Answer from the drawing. Dimensions are ordinates in mm from the lowest x, y and z of the part. Give positions to 0.01 mm unless a question says otherwise; leave off trailing zeros. Order: outer loops, then holes, each group sorted by start corner. A loop starts at its lowest first (then second) coordinate and runs counter-clockwise, first axis right, second up. Notation, with made-up numbers: (-27.75, -17.5) - (-1.75, -17.5) arc R16 cw to (-1.75, 8.5) - close; hole circle Ø3 at (35, -21). An arc over 180 degrees is marked (long way). Use a Markdown table: item, result. Add a question column.
1) Find section A-A, the plane x = 18. Determine the outline of the cut face in (y, z).
2) Find section D-D, the plane x = 13. Determine the outline of the cut face in (y, z).
3) A flat-ended cylindrical pin translates along its axis: pin 1 (14 mm diameter, centred on x = 13, z = 13.86, fed in from +Y). Find the tip coordinate at first contact, or state that the pin passes through.
4) Straight lines are drawn through the part: line 1 (Z direction, x = 9, y = 0.7) (1 decimal); line 2 (X direction, y = 1, z = 10.25) (1 decimal); line 3 (X direction, y = 0.65, z = 18) (1 decimal). For each, find the intervals that lie inside material, in ascending order.
5) Find section B-B, the plane z = 21.75. Determine the outline of the cut face in (x, y).
6) Find section C-C, the plane y = 0.4. Determine the outline of the cut face in (x, z) (1 decimal).
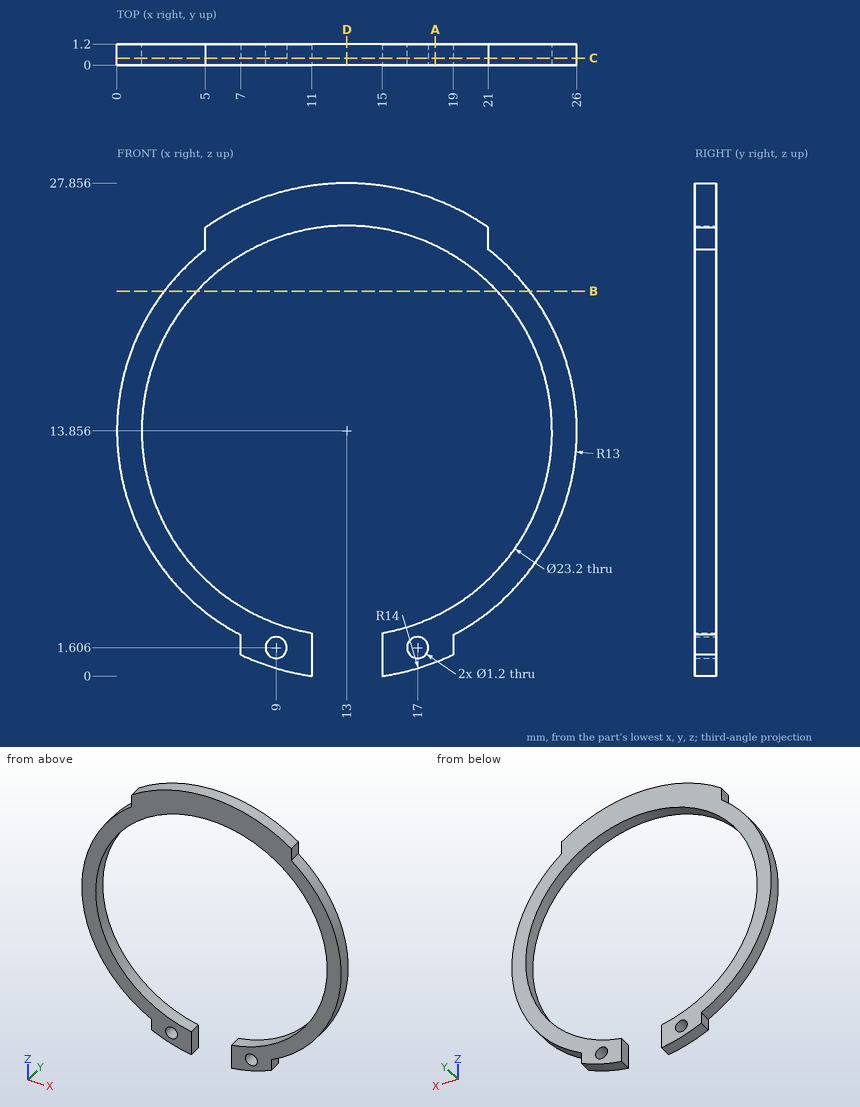
The answers:
| question | item | result |
|---|---|---|
| 1 | outline | (0, 0.78) - (1.2, 0.78) - (1.2, 3.39) - (0, 3.39) - close; (0, 24.32) - (1.2, 24.32) - (1.2, 26.93) - (0, 26.93) - close |
| 2 | outline | (0, 25.46) - (1.2, 25.46) - (1.2, 27.86) - (0, 27.86) - close |
| 3 | pin 1 | through |
| 4 | line 1 | 0.4 to 1, 2.2 to 3, 24.7 to 27.3 |
| 4 | line 2 | 0.5 to 2, 24 to 25.5 |
| 4 | line 3 | 0.7 to 2.2, 23.8 to 25.3 |
| 5 | outline | (2.67, 0) - (4.5, 0) - (4.5, 1.2) - (2.67, 1.2) - close; (21.5, 0) - (23.33, 0) - (23.33, 1.2) - (21.5, 1.2) - close |
| 6 | outline | (5, 24.1) arc R13 ccw to (7, 2.3) - (7, 1.2) arc R14 ccw to (11, 0) - (11, 2.4) arc R11.6 cw (long way) to (15, 2.4) - (15, 0) arc R14 ccw to (19, 1.2) - (19, 2.3) arc R13 ccw to (21, 24.1) - (21, 25.3) arc R14 ccw to (5, 25.3) - close; hole circle Ø1.2 at (9, 1.6); hole circle Ø1.2 at (17, 1.6) |
